```python
from build123d import *

# Parameters (mm, degrees)
BOSS_EXTRUDE1_DEPTH                = 8
TAP_DRILL_FOR_M2_5X0_45_TAP1_D     = 2.5
TAP_DRILL_FOR_M2_5X0_45_TAP1_DEPTH = 6.5


with BuildPart() as part:
    # Sketch1 → Boss-Extrude1 (new body)
    with BuildSketch(Plane(origin=(0, 0, 0), x_dir=(0, 0, -1), z_dir=(1, 0, 0))):
        with BuildLine():
            Line((-11.002014748, 0), (-15.002014748, 0))
            Line((-15.002014748, 0), (-15.002014748, -13.5))
            Line((-15.002014748, -13.5), (15.001777911, -13.5))
            Line((15.001777911, -13.5), (15.001777911, 0))
            Line((15.001777911, 0), (11.001777911, 0))
            Line((11.001777911, 0), (11, 0))
            ThreePointArc((11, 0), (0, -11), (-11, 0))
            Line((-11, 0), (-11.002014748, 0))
        make_face()
    extrude(amount=BOSS_EXTRUDE1_DEPTH)

    # Tap Drill for M2.5x0.45 Tap1
    with Locations(Plane(origin=(0, -13.5, 0), x_dir=(-1, 0, 0), z_dir=(0, -1, 0))):
        with Locations((-4, -12.502014748), (-4, 12.501777911)):
            Hole(TAP_DRILL_FOR_M2_5X0_45_TAP1_D / 2, depth=TAP_DRILL_FOR_M2_5X0_45_TAP1_DEPTH)


solid = part.part
```
Model file for the job. Use its own axes, mm. A direction names the side the tool comes from. Give positions to 0.01 mm unless a question says otherwise; leave off trailing zeros. Order: outer loops, then holes, each group sorted by start corner. A loop starts at its lowest first (then second) coordinate and runs counter-clockwise, first axis right, second up.
1) Pin check, flat tips, straight feed: pin 1 (1.5 mm diameter, centred on y = -8.5, z = -4.5, fed in from -X); pin 2 (2 mm diameter, centred on x = 4, z = 12.5, fed in from -Y). Stop position of each tip, or through.
2) Wall check: probe 1 along Z at (x, y) = (3.5, -7.5); probe 2 along Z at (x, y) = (4, -9); probe 3 along Y at (x, z) = (2, 0). Give the ranges that are in metal, low to high.
3) Saw through at B-B, the plane x = 4. Write the cut outline in (y, z), then the cut area to 3 significant figures.
4) Saw through at D-D, the plane z = 0. Write the cut outline in (x, y).
5) Saw through at C-C, the plane y = -4. Write the cut outline in (x, z), then the cut area to 3 significant figures.
6) Saw through at A-A, the plane y = -8.5. Write the cut outline in (x, z), then the cut area to 3 significant figures.
7) 3-axis set-ups, long thin cutter, end or side, ignore diameter. For faces 1 (the cylindrical face through (4, -11, 0)), 2 (the cylindrical face through (4.577, -10.204, -11.393)): which of +Z, -Z, +X, -X, +Y, -Y reach the whole face in a straight line?
8) Mould opens along X. For faces 3 (the flat face through (4, -13.5, 0)), 4 (the flat face through (0, -11.2, 0.2)), 5 (the cylindrical face through (5.155, -10.204, 12.981)) say: +X half, -X half, draft (parallel to the pull), parting line (faces both ways), or undercut.
Computed:
1. pin 1: passes through
1. pin 2: stops at y = -7
2. probe 1: z = -15 to -13.65, -11.36 to -8.05, 8.05 to 11.36, 13.65 to 15
2. probe 2: z = -15 to -13.75, -11.25 to -6.32, 6.32 to 11.25, 13.75 to 15
2. probe 3: y = -13.5 to -11
3. outline: (-13.5, -15) - (0, -15) - (0, -11) arc R11 cw to (0, 11) - (0, 15) - (-13.5, 15) - (-13.5, 13.75) - (-7, 13.75) - (-7, 11.25) - (-13.5, 11.25) - (-13.5, -11.25) - (-7, -11.25) - (-7, -13.75) - (-13.5, -13.75) - close
3. area: 182 mm2
4. outline: (0, -13.5) - (8, -13.5) - (8, -11) - (0, -11) - close
5. outline: (0, -15) - (8, -15) - (8, -10.25) - (0, -10.25) - close; (0, 10.25) - (8, 10.25) - (8, 15) - (0, 15) - close
5. area: 76.1 mm2
6. outline: (0, -15) - (8, -15) - (8, -6.98) - (0, -6.98) - close; (0, 6.98) - (8, 6.98) - (8, 15) - (0, 15) - close; hole circle Ø2.5 at (4, -12.5); hole circle Ø2.5 at (4, 12.5)
6. area: 118 mm2
7. face 1: +X, -X, +Y
7. face 2: -Y
8. face 3: draft
8. face 4: -X half
8. face 5: undercut
